Model file for the job. Use its own axes, mm. A direction names the side the tool comes from. Coordinates: 2 decimals unless noted, no trailing zeros. Order: outer loops, then holes, each group sorted by start corner. A loop starts at its lowest first (then second) coordinate and runs counter-clockwise, first axis right, second up. Notation, with made-up numbers: (61.25, -7.5) -> (96.25, -7.5) arc R19 cw to (96.25, 0.5) -> close; hole circle Ø2 at (71.5, 82.5). An arc over 180 degrees is marked (long way). Return JSON: item names as keys, results as strings. Group by question number.
1) Which spindle directions (+Z, -Z, +X, -X, +Y, -Y) get a long thin tool onto all of the face, cutting with end or side? Do faces 1 (the cylindrical face through (-6.08, 61.37, 8.77)), 2 (the flat face through (-44, 18, 12)), 3 (the flat face through (-20.689, 58, 36)). Say none if no direction does.
2) Cut at A-A (y = 33.5). Write the cut outline in (x, z).
3) Cut at D-D (x = -45). State how many separate pieces and enclosed holes the cut face has, and give its area (3 significant figures).
4) Flat gauge pins, fed straight in: pin 1 (15 mm diameter, centred on y = 56, z = 33.5, fed in from -X); pin 2 (5 mm diameter, centred on y = 62.5, z = 65, fed in from +X); pin 3 (2.5 mm diameter, centred on y = 4.5, z = 65, fed in from +X); pin 4 (18 mm diameter, centred on x = -36.5, y = 34, fed in from -Z). Where does each tip first touch, or does it go through?
5) Pull direction Z, two halves, no side cores. Call faces 4 (the flat face through (-53, 37, 6)), 5 (the cylindrical face through (-6.084, 4.773, 9.082)), 6 (the cylindrical face through (-18.734, 63.692, 68.863)): +Z half, -Z half, draft (parallel to the pull), parting line (faces both ways), or undercut.
6) Cut at C-C (z = 18.5). Write the cut outline in (x, y), and give its area (3 significant figures).
7) Cut at B-B (x = -26). Write the cut outline in (y, z).
8) Probe line 1 (Z direction, x = -46, y = 17); line 2 (Z direction, x = -5, y = 4.5); line 3 (Z direction, x = -4, y = 62). List the from-to ranges inside material, lowest first.
from build123d import *

# Parameters (mm, degrees)
SKETCH1_W             = 38
SKETCH1_H             = 67
BOSS_EXTRUDE1_DEPTH   = 72
SKETCH2_R             = 21
CUT_EXTRUDE1_DEPTH    = 6
CUT_EXTRUDE2_START    = -6
SKETCH3_R             = 21
CUT_EXTRUDE2_DEPTH    = 6
SKETCH4_W             = 50.811271485
SKETCH4_H             = 48
CUT_EXTRUDE3_DEPTH    = 122.594613368
SKETCH6_R             = 15
CUT_EXTRUDE4_DEPTH    = 200
FILLET2_R             = 11
SKETCH10_W            = 47
SKETCH10_H            = 29.40683467
CUT_EXTRUDE7_DEPTH    = 82
CUT_EXTRUDE10_REACH   = 123.595
M5_TAPPED_HOLE1_D     = 4.2
M5_TAPPED_HOLE1_DEPTH = 12
M5_TAPPED_HOLE1_TIP   = 1.2618073
SKETCH13_W            = 0.5
SKETCH13_H            = 18.5
CUT_EXTRUDE11_DEPTH   = 111.701333822


with BuildPart() as part:
    # Sketch1 → Boss-Extrude1 (new body)
    with BuildSketch(Plane.XY):
        with Locations((-19, 33.5)):
            Rectangle(SKETCH1_W, SKETCH1_H)
        with BuildLine():
            Line((-38, 0), (-38, 67))
            ThreePointArc((-38, 67), (-71.5, 33.5), (-38, 0))
        make_face()
    extrude(amount=BOSS_EXTRUDE1_DEPTH)

    # Sketch2 → Cut-Extrude1 (cut)
    with BuildSketch(Plane(origin=(0, 0, 0), x_dir=(-1, 0, 0), z_dir=(0, 0, -1))):
        with Locations((38, 33.5)):
            Circle(SKETCH2_R)
    extrude(amount=-CUT_EXTRUDE1_DEPTH, mode=Mode.SUBTRACT)

    # Sketch3 → Cut-Extrude2 (cut)
    with BuildSketch(Plane.XY.offset(72).offset(CUT_EXTRUDE2_START)):
        with Locations(Location((-38, 33.5, 0), (0, 0, 180))):
            Circle(SKETCH3_R)
    extrude(amount=CUT_EXTRUDE2_DEPTH, mode=Mode.SUBTRACT)

    # Sketch4 → Cut-Extrude3 (cut, through all)
    with BuildSketch(Plane.XZ):
        with Locations((-46.094364258, 36)):
            Rectangle(SKETCH4_W, SKETCH4_H)
    extrude(amount=-CUT_EXTRUDE3_DEPTH, mode=Mode.SUBTRACT)

    # Sketch6 → Cut-Extrude4 (cut)
    with BuildSketch(Plane(origin=(0, 0, 0), x_dir=(-1, 0, 0), z_dir=(0, 0, -1))):
        with Locations((38, 33.5)):
            Circle(SKETCH6_R)
    extrude(amount=-CUT_EXTRUDE4_DEPTH, mode=Mode.SUBTRACT)

    # Fillet2
    fillet2_edges = [part.edges().sort_by_distance(p)[0] for p in [
        (-19, 67, 72),
        (-71.5, 33.5, 72),
        (-19, 0, 72),
        (-19, 0, 0),
        (-71.5, 33.5, 0),
        (-19, 67, 0),
    ]]
    fillet(fillet2_edges, radius=FILLET2_R)

    # Sketch10 → Cut-Extrude7 (cut)
    with BuildSketch(Plane(origin=(0, 0, 0), x_dir=(0, 0, -1), z_dir=(1, 0, 0))):
        with Locations((-36, 14.703417335)):
            Rectangle(SKETCH10_W, SKETCH10_H)
    extrude(amount=-CUT_EXTRUDE7_DEPTH, mode=Mode.SUBTRACT)

    # Sketch11 → Cut-Extrude10 (cut, up to next)
    with BuildSketch(Plane.XY.offset(72), mode=Mode.PRIVATE) as cut_extrude10_sk1:
        with BuildLine():
            Line((-38, 48.5), (-38, 33.5))
            Line((-38, 33.5), (-17, 33.5))
            ThreePointArc((-17, 33.5), (-18.639786835, 41.635241005), (-23.303061543, 48.5))
            Line((-23.303061543, 48.5), (-38, 48.5))
        make_face()
    cut_extrude10_tool1 = extrude(cut_extrude10_sk1.sketch, amount=-CUT_EXTRUDE10_REACH, mode=Mode.PRIVATE) & part.part
    # Sketch11 → Cut-Extrude10 (cut, up to next)
    with BuildSketch(Plane.XY.offset(72), mode=Mode.PRIVATE) as cut_extrude10_sk2:
        with BuildLine():
            ThreePointArc((-23.303061543, 48.5), (-18.639786835, 41.635241005), (-17, 33.5))
            Line((-17, 33.5), (0, 33.5))
            Line((0, 33.5), (0, 48.5))
            Line((0, 48.5), (-23.303061543, 48.5))
        make_face()
    cut_extrude10_tool2 = extrude(cut_extrude10_sk2.sketch, amount=-CUT_EXTRUDE10_REACH, mode=Mode.PRIVATE) & part.part
    # Sketch11 → Cut-Extrude10 (cut, up to next)
    with BuildSketch(Plane.XY.offset(72), mode=Mode.PRIVATE) as cut_extrude10_sk3:
        with BuildLine():
            Line((0, 33.5), (-17, 33.5))
            ThreePointArc((-17, 33.5), (-18.639786835, 25.364758995), (-23.303061543, 18.5))
            Line((-23.303061543, 18.5), (0, 18.5))
            Line((0, 18.5), (0, 33.5))
        make_face()
    cut_extrude10_tool3 = extrude(cut_extrude10_sk3.sketch, amount=-CUT_EXTRUDE10_REACH, mode=Mode.PRIVATE) & part.part
    # Sketch11 → Cut-Extrude10 (cut, up to next)
    with BuildSketch(Plane.XY.offset(72), mode=Mode.PRIVATE) as cut_extrude10_sk4:
        with BuildLine():
            Line((-17, 33.5), (-38, 33.5))
            Line((-38, 33.5), (-38, 18.5))
            Line((-38, 18.5), (-23.303061543, 18.5))
            ThreePointArc((-23.303061543, 18.5), (-18.639786835, 25.364758995), (-17, 33.5))
        make_face()
    cut_extrude10_tool4 = extrude(cut_extrude10_sk4.sketch, amount=-CUT_EXTRUDE10_REACH, mode=Mode.PRIVATE) & part.part
    add(cut_extrude10_tool1.solids().sort_by_distance((-28.39059, 40.602283, 72))[0], mode=Mode.SUBTRACT)
    add(cut_extrude10_tool2.solids().sort_by_distance((-9.565982, 41.399556, 72))[0], mode=Mode.SUBTRACT)
    add(cut_extrude10_tool3.solids().sort_by_distance((-9.565982, 25.600444, 72))[0], mode=Mode.SUBTRACT)
    add(cut_extrude10_tool4.solids().sort_by_distance((-28.39059, 26.397717, 72))[0], mode=Mode.SUBTRACT)

    # M5 Tapped Hole1
    with Locations(Plane(origin=(0, 62.5, 65), x_dir=(0, 1, 0), z_dir=(1, 0, 0))):
        with Locations((0, 0), (0, -58), (-58, -58), (-58, 0)):
            Hole(M5_TAPPED_HOLE1_D / 2, depth=M5_TAPPED_HOLE1_DEPTH)
            with Locations((0, 0, -(M5_TAPPED_HOLE1_DEPTH + M5_TAPPED_HOLE1_TIP / 2))):  # 118° drill point
                Cone(0, M5_TAPPED_HOLE1_D / 2, M5_TAPPED_HOLE1_TIP, mode=Mode.SUBTRACT)

    # Sketch13 → Cut-Extrude11 (cut, through all)
    with BuildSketch(Plane.ZY.offset(20.688728515)):
        with Locations((59.75, 9.25)):
            Rectangle(SKETCH13_W, SKETCH13_H)
        with Locations((12.25, 9.25)):
            Rectangle(SKETCH13_W, SKETCH13_H)
    extrude(amount=-CUT_EXTRUDE11_DEPTH, mode=Mode.SUBTRACT)


solid = part.part
Answers below:
{
 "1": {"face 1": "+X", "face 2": "-X, -Y", "face 3": "-X, +Y, -Y"},
 "2": {"outline": "(-71.5, 11) arc R11 ccw to (-60.5, 0) -> (-59, 0) -> (-59, 6) -> (-53, 6) -> (-53, 12) -> (-71.5, 12) -> close; (-71.5, 60) -> (-53, 60) -> (-53, 66) -> (-59, 66) -> (-59, 72) -> (-60.5, 72) arc R11 ccw to (-71.5, 61) -> close"},
 "3": {"separate pieces": "4", "enclosed holes": "0", "area": "672 mm^2"},
 "4": {"pin 1": "stops at x = -20.69", "pin 2": "stops at x = 0", "pin 3": "stops at x = -12.51", "pin 4": "passes through"},
 "5": {"face 4": "-Z half", "face 5": "undercut", "face 6": "+Z half"},
 "6": {"outline": "(-20.69, 48.5) -> (0, 48.5) -> (0, 67) -> (-20.69, 67) -> close", "area": "383 mm^2"},
 "7": {"outline": "(0, 11) arc R11 ccw to (11, 0) -> (16.27, 0) -> (16.27, 6) -> (18.5, 6) -> (18.5, 12) -> (0, 12) -> close; (0, 60) -> (18.5, 60) -> (18.5, 66) -> (16.27, 66) -> (16.27, 72) -> (11, 72) arc R11 ccw to (0, 61) -> close; (48.5, 6) -> (50.73, 6) -> (50.73, 0) -> (56, 0) arc R11 ccw to (67, 11) -> (67, 12) -> (48.5, 12) -> close; (48.5, 60) -> (67, 60) -> (67, 61) arc R11 ccw to (56, 72) -> (50.73, 72) -> (50.73, 66) -> (48.5, 66) -> close"},
 "8": {"line 1": "z = 6 to 12, 60 to 66", "line 2": "z = 2.13 to 4.9, 9.1 to 12, 60 to 62.9, 67.1 to 69.87", "line 3": "z = 1.78 to 4.96, 9.04 to 62.96, 67.04 to 70.22"}
}
